Source: CAD feature listing. Evaluate the final solid. Frame: model axes, mm. A direction names the side the tool comes from. Give positions to 0.01 mm unless a question says otherwise; leave off trailing zeros. Loops run counter-clockwise (first coordinate to the right, second up) from the corner with the lowest first, then second, coordinate; pieces in that order, holes last. Notation, with made-up numbers: M -26,82.25 L 10,82.25 A30 cw 10,113.25 Z; hole C 81,71.5 d3. An arc over 180 degrees is marked long. Write item = value, one per line.
Autodesk Inventor part; units mm, degrees
ref_plane "YZ Plane" through (0, 0, 0) normal (1, 0, 0) x (0, 1, 0)
ref_plane "XZ Plane" through (0, 0, 0) normal (0, 1, 0) x (-1, 0, 0)
ref_plane "XY Plane" through (0, 0, 0) normal (0, 0, 1) x (1, 0, 0)
sketch "Skizze1" plane through (0, 0, 0) normal (0, 0, 1) x (1, 0, 0)
  circle A0 centre (4.9, 12.1) radius 0.455
  circle A1 centre (4.9, 12.1) radius 0.7
  line L0 (6.3, 10.875) -> (6.3, 12.1)
  line L1 (0, 15) -> (7, 15)
  line L2 (7, 15) -> (7, 13.75)
  line L3 (7, 13.75) -> (1.75, 13.75)
  line L4 (0, 0) -> (9.5856, 0)
  line L5 (0, 15) -> (0, 12.1)
  line L6 (0, 12.1) -> (1.75, 11.75)
  line L7 (1.75, 11.75) -> (4.9, 10)
  line L8 (4.9, 10) -> (6.3, 10.875)
  line L9 (4.9, 10) -> (0, 10) construction
  line L10 (0, 18) -> (0, -3)
  line L11 (-1.9171, 0) -> (11.5027, 0)
  line L12 (4.2, 12.1) -> (1.75, 12.59)
  line L13 (1.75, 12.59) -> (1.75, 13.75)
  line L14 (6.3, 12.1) -> (5.6, 12.1)
  dimension "d0" = 30
  dimension "d1" = 21.75
  dimension "d2" = 1.25
  dimension "d3" = 0.91
  dimension "d4" = 1.4
  dimension "d5" = 20
  dimension "d6" = 23.5
  dimension "d7" = 24.2
  dimension "d8" = 4.9
  dimension "d9" = 6.3
  dimension "d10" = 7
  dimension "d12" = 1.75
revolve "Körper" add sketch "Skizze1" angle 360 about axis through (0, 0, 0) along (1, 0, 0) contours L14 L0 L8 L7 L6 L5 L1 L2 L3 L13 L12 A1
revolve "Feder1" add sketch "Skizze1" angle 360 about axis through (0, 0, 0) along (1, 0, 0) contours A0 | A1
fillet "Rundung1" radius 0.3 3 edges at (7, -15, 0) (1.75, -13.75, 0) (0, -15, 0)
equation "\"d0\" = SD2"
equation "\"d1\" = ABDM"
equation "\"d3\" = SPDI"
equation "\"d4\" = SPDA"
equation "\"d5\" = NND"
equation "\"d6\" = TKDM"
equation "\"d7\" = HLDM"
equation "\"d8\" = SPDST"
equation "\"d9\" = SDI"
equation "\"d10\" = SWDT"
equation "\"d12\" = SD"
equation "\"d11\" = RR"
equation "\"SD2\" = 30"
equation "\"SWDT\" = 7"
equation "\"RR\" = 0.3"
equation "\"SD\" = 1.75"
equation "\"NND\" = 20"
equation "\"SPDA\" = 1.4"
equation "\"SPDI\" = 0.91"
equation "\"TKDM\" = 23.5"
equation "\"HLDM\" = 24.2"
equation "\"ABDM\" = 21.75"
equation "\"SDI\" = 6.3"
equation "\"SPDST\" = 4.9"
equation "\"LAB\" = 0.35"
properties part number "DIN 3760 - A - 20 x 30 x 7 - NBR" material "Gummi"
1. Material intervals for probe 1 along Z at (x, y) = (3.25, 1); probe 2 along Y at (x, z) = (4.75, -9); probe 3 along Z at (x, y) = (2.25, 8.5), sorted ascending. Write a range as from..to.
Derived:
probe_1 = -14.97..-13.71, -12.25..-10.87, 10.87..12.25, 13.71..14.97
probe_2 = -12..-10.4, -9.08..-4.55, 4.55..9.08, 10.4..12
probe_3 = -12.36..-10.81, -9.15..-7.7, 7.7..9.15, 10.81..12.36
2. Pull-direction query (Z, two-part tool) for faces 1 (the cylindrical face through (4.49, -2.981, 13.423)), 2 (the flat face through (7, 10, -10)), 3 (the cylindrical face through (3.545, -14.985, 0.66)); classes: +Z half, -Z half, draft (parallel to the pull), parting line (faces both ways), or undercut.
Derived:
face_1 = undercut
face_2 = draft
face_3 = parting line
3. Reachability of faces 4 (the cylindrical face through (5.95, 11.18, 4.63)), 5 (the flat face through (1.75, 8, -10)), 6 (the flat face through (0, -11, 6)) from +Z, -Z, +X, -X, +Y, -Y: full face, straight path, thin tool, end or side. Return the list, or none.
Derived:
face_4 = +X
face_5 = none
face_6 = +Z, -Z, -X, +Y, -Y
4. Cut plane C-C, the plane x = 2.5. Return the cut outline in (y, z).
Derived:
outline = C 0,0 d30; C 0,0 d24.88; hole C 0,0 d27.5; hole C 0,0 d22.67
5. First-contact query: pin 1 Ø1 at (x, y) = (2, 2.5) entering from -Z; pin 2 Ø1.5 at (x, y) = (4.5, -6.5) entering from -Z; pin 3 Ø12 at (y, z) = (-7.5, 9) entering from +X; pin 4 Ø2 at (x, y) = (1, -8) entering from -Z. Flat tips, straight axial feed; report the tip coordinate or a pass-through.
Derived:
pin_1 = -14.87
pin_2 = -13.85
pin_3 = 7
pin_4 = -13.27
